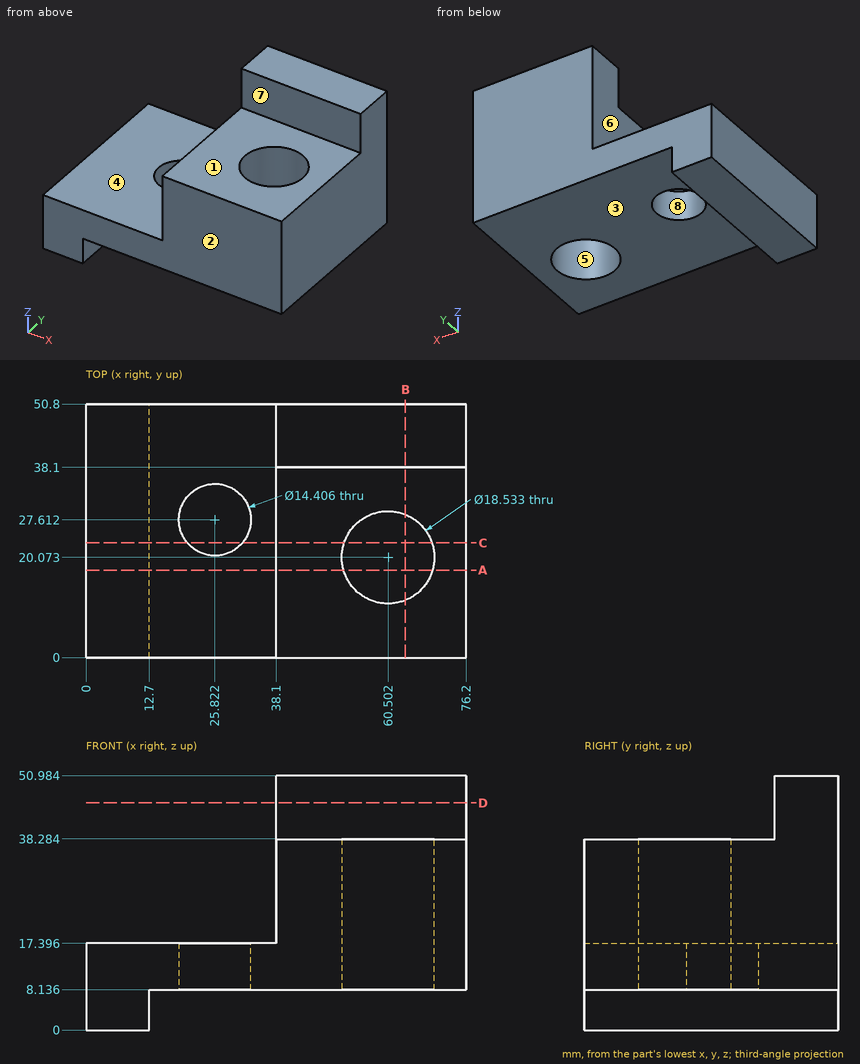
Here's the drawing with two shaded views (mm, measured from the low corner). I have some questions. A direction names the side the tool comes from. Coordinates: 2 decimals unless noted, no trailing zeros. Order: outer loops, then holes, each group sorted by start corner. A loop starts at its lowest first (then second) coordinate and runs counter-clockwise, first axis right, second up. Notation, with made-up numbers: M 82,41 L 111,41 A12 ccw 111,45 Z; hole C -25.5,48.5 d4. An arc over 180 degrees is marked long. Answer as CSV lines item,"result".
Item 1: On a 3-axis mill with a long thin cutter (end or side, diameter ignored), from which of +Z, -Z, +X, -X, +Y, -Y can I reach the whole of each face in a straight line? I mean the marked faces 1, 2, 3 and 4. Say none if no direction works.
Results found:
face 1,"+Z, +X, -X, -Y"
face 2,"+Z, -Z, +X, -X, -Y"
face 3,"-Z, +X, +Y, -Y"
face 4,"+Z, -X, +Y, -Y"
Item 2: Imagine slicing it at B-B on x = 64. Write out the boundary of the cut face in (y, z), plus the area to 3 significant figures.
Results found:
outline,"M 0,8.14 L 11.49,8.14 L 11.49,38.28 L 0,38.28 Z; M 28.65,8.14 L 50.8,8.14 L 50.8,50.98 L 38.1,50.98 L 38.1,38.28 L 28.65,38.28 Z"
area,"1,180 mm2"
Item 3: Imagine slicing it at A-A on y = 17.5. Write out the boundary of the cut face in (x, z) (1 decimal).
Results found:
outline,"M 0,0 L 12.7,0 L 12.7,8.1 L 51.6,8.1 L 51.6,38.3 L 38.1,38.3 L 38.1,17.4 L 0,17.4 Z; M 69.4,8.1 L 76.2,8.1 L 76.2,38.3 L 69.4,38.3 Z"
Item 4: We'd pull the mould along Y, two halves only. Please class the marked faces 5, 6, 7 and 8: +Y half, -Y half, draft (parallel to the pull), parting line (faces both ways), or undercut.
Results found:
face 5,"undercut"
face 6,"draft"
face 7,"-Y half"
face 8,"undercut"
Item 5: For pin 1 (2 mm diameter, centred on x = 29, z = 8, fed in from +Y); pin 2 (4 mm diameter, centred on y = 31, z = 37.5, fed in from -X); pin 3 (8 mm diameter, centred on x = 10.5, y = 23.5, fed in from +Z); pin 4 (2 mm diameter, centred on x = 21.5, y = 20, fed in from -Z), each with a flat end and sliding along its axis, tell me the tip position at first contact or that it passes through.
Results found:
pin 1,"y = 50.8"
pin 2,"x = 38.1"
pin 3,"z = 17.4"
pin 4,"z = 8.14"
Item 6: Imagine slicing it at D-D on z = 45.5. Write out the boundary of the cut face in (x, y).
Results found:
outline,"M 38.1,38.1 L 76.2,38.1 L 76.2,50.8 L 38.1,50.8 Z"
Item 7: Imagine slicing it at C-C on y = 23. Write out the boundary of the cut face in (x, z) (1 decimal), plus the area to 3 significant figures.
Results found:
outline,"M 0,0 L 12.7,0 L 12.7,8.1 L 20.3,8.1 L 20.3,17.4 L 0,17.4 Z; M 31.4,8.1 L 51.7,8.1 L 51.7,38.3 L 38.1,38.3 L 38.1,17.4 L 31.4,17.4 Z; M 69.3,8.1 L 76.2,8.1 L 76.2,38.3 L 69.3,38.3 Z"
area,"972 mm2"
Item 8: If I drill on line 1 (X direction, y = 20.5, z = 29) (1 decimal); line 2 (Z direction, x = 28, y = 48.5); line 3 (Z direction, x = 4.5, y = 4), over which ranges is the centre line in solid material (lowest first)?
Results found:
line 1,"38.1 to 51.2, 69.8 to 76.2"
line 2,"8.14 to 17.4"
line 3,"0 to 17.4"
